Design review of the part built by this model. Coordinates are the model's own, in mm. Round coordinates to 2 decimals unless told otherwise and drop trailing zeros. Loops run counter-clockwise (first coordinate to the right, second up) from the corner with the lowest first, then second, coordinate; pieces in that order, holes last. Notation, with made-up numbers: (-19, -17) - (34, -17) arc R25 ccw to (34, 16) - close; hole circle Ø8 at (29.25, 4.25). An arc over 180 degrees is marked (long way). Answer as CSV lines item,"result". Start each with the question number.
(1) Consider section B-B (x = 48). Give the boundary of the cut face in (y, z).
(2) Consider section A-A (y = 0). Give the boundary of the cut face in (x, z), and give its area (3 significant figures).
(3) Wall thickness on L1, parallel to Y at x = 63.5, z = -4.9; L2, parallel to X at y = 0.5, z = -4.25; L3, parallel to Z at x = -17.5, y = 0.9: over which ranges is each line inside the solid? List them lowest first.
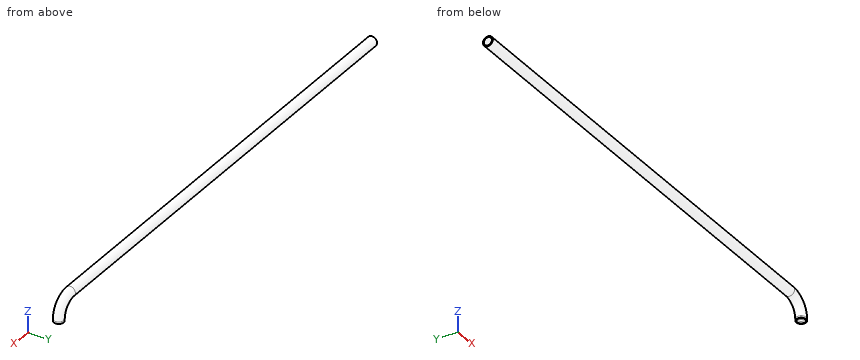
from build123d import *

# Parameters (mm, degrees)
SKIZZE1_R                       = 1.25
SKIZZE1_R_2                     = 1
AUFSATZ_LINEAR_AUSTRAGEN1_DEPTH = 58.5
SKIZZE2_R                       = 1.25
SKIZZE2_R_2                     = 1


with BuildPart() as part:
    # Skizze1 → Aufsatz-Linear austragen1 (new, symmetric)
    with BuildSketch(Plane(origin=(0, 0, 0), x_dir=(0, 0, -1), z_dir=(1, 0, 0))):
        Circle(SKIZZE1_R)
        Circle(SKIZZE1_R_2, mode=Mode.SUBTRACT)
    extrude(amount=AUFSATZ_LINEAR_AUSTRAGEN1_DEPTH, both=True)

    # Austragung1: sweep along a path in Skizze3
    with BuildLine(Plane(origin=(0, 0, 0), x_dir=(1, 0, 0), z_dir=(0, 1, 0))) as austragung1_path:
        Line((58.5, 0), (59, 0))
        ThreePointArc((59, 0), (62.181980515, 1.318019485), (63.5, 4.5))
        Line((63.5, 4.5), (63.5, 5))
    # Skizze2 → Austragung1 (sweep)
    with BuildSketch(Plane(origin=(58.5, 0, 0), x_dir=(0, 0, -1), z_dir=(1, 0, 0))):
        Circle(SKIZZE2_R)
        Circle(SKIZZE2_R_2, mode=Mode.SUBTRACT)
    sweep(path=austragung1_path.line)


solid = part.part
Determined:
1,outline,"circle Ø2.5 at (0, 0); hole circle Ø2 at (0, 0)"
2,outline,"(-58.5, -1.25) - (59, -1.25) arc R3.25 cw to (62.25, -4.5) - (62.25, -5) - (62.5, -5) - (62.5, -4.5) arc R3.5 ccw to (59, -1) - (-58.5, -1) - close; (-58.5, 1) - (59, 1) arc R5.5 cw to (64.5, -4.5) - (64.5, -5) - (64.75, -5) - (64.75, -4.5) arc R5.75 ccw to (59, 1.25) - (-58.5, 1.25) - close"
2,area,"62.5 mm^2"
3,L1,"y = -1.25 to -1, 1 to 1.25"
3,L2,"x = 62.35 to 62.63, 64.36 to 64.64"
3,L3,"z = -0.87 to -0.44, 0.44 to 0.87"
